Print and shaded views of the part. All mm, measured from the part's lowest x, y and z. A direction names the side the tool comes from. Round coordinates to 2 decimals unless told otherwise and drop trailing zeros. Order: outer loops, then holes, each group sorted by start corner. A loop starts at its lowest first (then second) coordinate and runs counter-clockwise, first axis right, second up. Notation, with made-up numbers: (19.5, -37) -> (41.5, -37) arc R20 ccw to (41.5, -14) -> close; hole circle Ø11 at (-11, 16). An arc over 180 degrees is marked (long way). Answer as CSV lines item,"result".
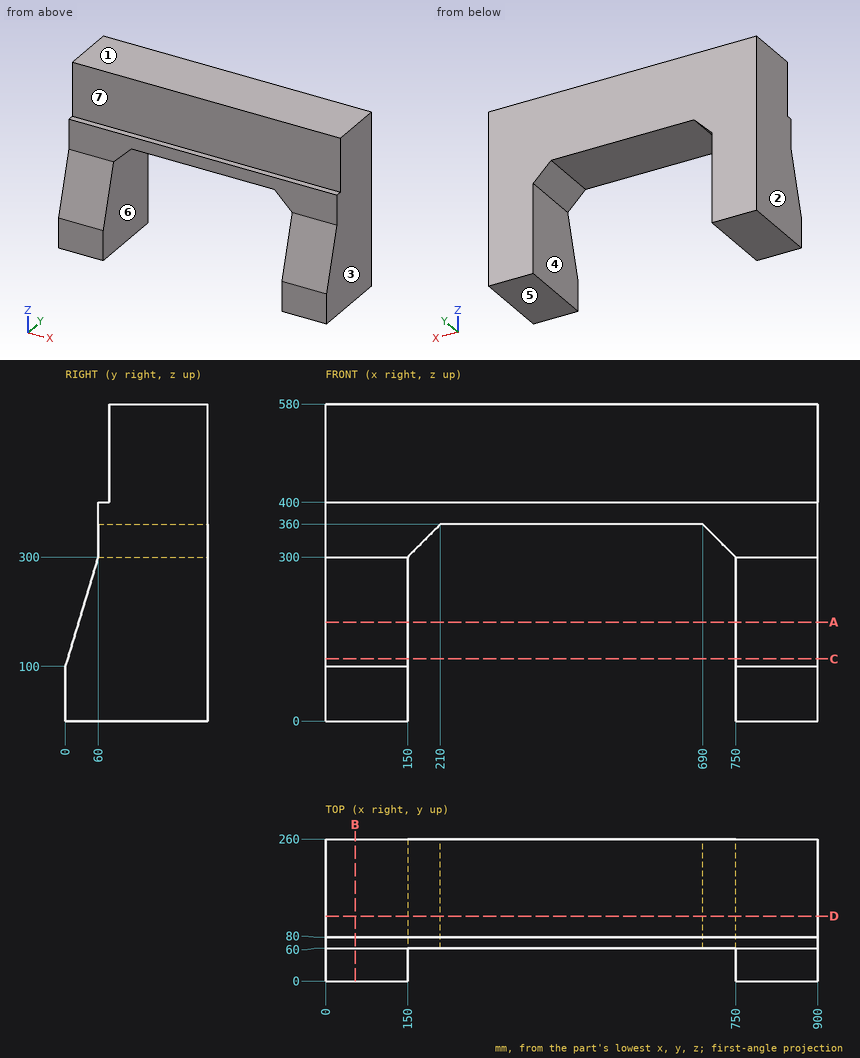
Q1. Saw through at D-D (y = 119). Write the cut outline in (x, z).
Checks:
outline,"(0, 0) -> (150, 0) -> (150, 300) -> (210, 360) -> (690, 360) -> (750, 300) -> (750, 0) -> (900, 0) -> (900, 580) -> (0, 580) -> close"
Q2. Flat gauge pin, fed straight in: pin 1 (3 mm diameter, centred on x = 574.5, y = 175, fed in from -Z). Where does the tip first touch, or does it go through?
Checks:
pin 1,"z = 360"
Q3. Mould opens along X. For the marked faces 1, 2, 3 and 4 say: +X half, -X half, draft (parallel to the pull), parting line (faces both ways), or undercut.
Checks:
face 1,"draft"
face 2,"-X half"
face 3,"+X half"
face 4,"undercut"
Q4. Saw through at B-B (x = 54). Write the cut outline in (y, z).
Checks:
outline,"(0, 0) -> (260, 0) -> (260, 580) -> (80, 580) -> (80, 400) -> (60, 400) -> (60, 300) -> (0, 100) -> close"
Q5. Saw through at A-A (z = 181). Write the cut outline in (x, y), plus the area to 3 significant figures.
Checks:
outline,"(0, 24.3) -> (150, 24.3) -> (150, 260) -> (0, 260) -> close; (750, 24.3) -> (900, 24.3) -> (900, 260) -> (750, 260) -> close"
area,"70,700 mm²"
Q6. Tool access for the marked faces 5, 6 and 7: list every direction of +Z, -Z, +X, -X, +Y, -Y with a clear straight run to the whole face (end or side of a thin tool).
Checks:
face 5,"-Z, +X, -X, +Y, -Y"
face 6,"-Z, +Y, -Y"
face 7,"+Z, +X, -X, -Y"
Q7. Saw through at C-C (z = 113.5). Write the cut outline in (x, y), plus the area to 3 significant figures.
Checks:
outline,"(0, 4.05) -> (150, 4.05) -> (150, 260) -> (0, 260) -> close; (750, 4.05) -> (900, 4.05) -> (900, 260) -> (750, 260) -> close"
area,"76,800 mm²"
Q8. Wall check: L1, parallel to X at y = 200, z = 203; L2, parallel to Z at x = 307.5, y = 242.5; L3, parallel to Y at x = 144, z = 406.5. Give the ranges that are in metal, low to high. Write a range as [from, to].
Checks:
L1,"[0, 150], [750, 900]"
L2,"[360, 580]"
L3,"[80, 260]"
